Source: CAD feature listing. Evaluate the final solid. Frame: model axes, mm. A direction names the side the tool comes from. Coordinates: 2 decimals unless noted, no trailing zeros. Order: outer loops, then holes, each group sorted by start corner. A loop starts at its lowest first (then second) coordinate and runs counter-clockwise, first axis right, second up.
Item 1: Reachability of faces 5 (the flat face through (2, 8.3, -6)), 6 (the cylindrical face through (4.57, 10.582, -7.167)), 7 (the flat face through (0, 9.3, 0)) from +Z, -Z, +X, -X, +Y, -Y: full face, straight path, thin tool, end or side. Return the list, or none.
Item 2: Section A-A on z = 0. Return the cut outline in (x, y), then the cut area to 3 significant figures.
Item 3: Section C-C on y = 10.5. Return the cut outline in (x, z), then the cut area to 3 significant figures.
Item 4: Section B-B on x = 0. Return the cut outline in (y, z), then the cut area to 3 significant figures.
Item 5: Mould query, pull axis X, two halves, no side actions, for faces 1 (the flat face through (0, 0, 0)), 2 (the cylindrical face through (-6, 4, 0)), 3 (the cylindrical face through (-0.29, 10.31, -2.23)), 4 (the cylindrical face through (-2.579, 11.959, 1.978)). Classes: released by +X, released by -X, zero draft, split by the parting line, or undercut.
Item 6: Ray query, line 1 (X direction, y = 10.45, z = 0); line 2 (Y direction, x = 6.25, z = -5). Return the intervals inside material, ascending.
Item 7: Contact query for flat-ended pins moving along their axis: P1, Ø3.5, axis at x = 0.5, z = -0.5, coming from the +Y side; P2, Ø4, axis at x = 0, z = 0, coming from the +Y side; P3, Ø4, axis at y = 9.5, z = -2.5, coming from the +X side; P4, Ø8.5, axis at x = -1.5, z = 3, coming from the -Y side. Output: stop coordinate, or through.
Item 8: Section D-D on y = 5.75. Return the cut outline in (x, z), then the cut area to 3 significant figures.
from build123d import *

# Parameters (mm, degrees)
SKETCH1_R           = 7
BOSS_EXTRUDE1_DEPTH = 12.8
SKETCH2_OUTSIDE_W   = 20.716
SKETCH2_OUTSIDE_H   = 20.716
SKETCH2_OUTSIDE_R   = 6
CUT_EXTRUDE1_DEPTH  = 13.8
SKETCH3_R           = 3.25
CUT_EXTRUDE2_DEPTH  = 1.5
SKETCH4_R           = 2.25
CUT_EXTRUDE3_DEPTH  = 2
CHAMFER1_SIZE       = 0.2
SKETCH_1_R          = 8.5
SKETCH_1_R_2        = 5.212411732
EXTRUDE_1_DEPTH     = 4.5


with BuildPart() as part:
    # Sketch1 → Boss-Extrude1 (new body)
    with BuildSketch(Plane(origin=(0, 0, 0), x_dir=(1, 0, 0), z_dir=(0, 1, 0))):
        Circle(SKETCH1_R)
    extrude(amount=BOSS_EXTRUDE1_DEPTH)

    # Sketch2 outside → Cut-Extrude1 (cut, through all)
    with BuildSketch(Plane.XZ):
        Rectangle(SKETCH2_OUTSIDE_W, SKETCH2_OUTSIDE_H)
        Circle(SKETCH2_OUTSIDE_R, mode=Mode.SUBTRACT)
    extrude(amount=-CUT_EXTRUDE1_DEPTH, mode=Mode.SUBTRACT)

    # Sketch3 → Cut-Extrude2 (cut)
    with BuildSketch(Plane(origin=(0, 12.8, 0), x_dir=(1, 0, 0), z_dir=(0, 1, 0))):
        Circle(SKETCH3_R)
    extrude(amount=-CUT_EXTRUDE2_DEPTH, mode=Mode.SUBTRACT)

    # Sketch4 → Cut-Extrude3 (cut)
    with BuildSketch(Plane(origin=(0, 11.3, 0), x_dir=(1, 0, 0), z_dir=(0, 1, 0))):
        Circle(SKETCH4_R)
    extrude(amount=-CUT_EXTRUDE3_DEPTH, mode=Mode.SUBTRACT)

    # Chamfer1
    chamfer1_edges = [part.edges().sort_by_distance(p)[0] for p in [
        (-3.25, 12.8, 0),
    ]]
    chamfer(chamfer1_edges, length=CHAMFER1_SIZE)

    # ｽｹｯﾁ1 → ﾎﾞｽ - 押し出し1 (add)
    with BuildSketch(Plane(origin=(0, 12.8, 0), x_dir=(1, 0, 0), z_dir=(0, 1, 0))):
        Circle(SKETCH_1_R)
        Circle(SKETCH_1_R_2, mode=Mode.SUBTRACT)
    extrude(amount=-EXTRUDE_1_DEPTH)


solid = part.part
Answer list:
1. face 5: -Y
1. face 6: +Y, -Y
1. face 7: +Y
2. outline: (-8.5, 8.3) - (-6, 8.3) - (-6, 0) - (6, 0) - (6, 8.3) - (8.5, 8.3) - (8.5, 12.8) - (3.45, 12.8) - (3.25, 12.6) - (3.25, 11.3) - (2.25, 11.3) - (2.25, 9.3) - (-2.25, 9.3) - (-2.25, 11.3) - (-3.25, 11.3) - (-3.25, 12.6) - (-3.45, 12.8) - (-8.5, 12.8) - close
2. area: 157 mm2
3. outline: circle Ø17 at (0, 0); hole circle Ø4.5 at (0, 0)
3. area: 211 mm2
4. outline: (0, -6) - (8.3, -6) - (8.3, -8.5) - (12.8, -8.5) - (12.8, -3.45) - (12.6, -3.25) - (11.3, -3.25) - (11.3, -2.25) - (9.3, -2.25) - (9.3, 2.25) - (11.3, 2.25) - (11.3, 3.25) - (12.6, 3.25) - (12.8, 3.45) - (12.8, 8.5) - (8.3, 8.5) - (8.3, 6) - (0, 6) - close
4. area: 157 mm2
5. face 1: zero draft
5. face 2: split by the parting line
5. face 3: undercut
5. face 4: undercut
6. line 1: x = -8.5 to -2.25, 2.25 to 8.5
6. line 2: y = 8.3 to 12.8
7. P1: stops at y = 11.3
7. P2: stops at y = 9.3
7. P3: stops at x = 8.49
7. P4: stops at y = 0
8. outline: circle Ø12 at (0, 0)
8. area: 113 mm2
